```python
from build123d import *

# Parameters (mm, degrees)
BOSS_EXTRUDE1_DEPTH      = 15.875
BOSS_EXTRUDE1_DEPTH_BACK = 15.875


with BuildPart() as part:
    # Sketch2 → Boss-Extrude1 (new, two sides: drawn at the far end of the back side and taken through both)
    with BuildSketch(Plane(origin=(0, 0, 0), x_dir=(1, 0, 0), z_dir=(0, 1, 0)).offset(-BOSS_EXTRUDE1_DEPTH_BACK)):
        Polygon((-171.45, 88.9), (-171.45, -88.9), (-165.1, -88.9), (-165.1, -79.375), (-161.925, -79.375), (-161.925, 25.4), (-161.925, 34.925), (-161.925, 79.375), (-165.1, 79.375), (-165.1, 88.9), align=None)
    extrude(amount=BOSS_EXTRUDE1_DEPTH + BOSS_EXTRUDE1_DEPTH_BACK)


solid = part.part
```
Can you work these out from the model? Positions are in its coordinate system, mm. A direction names the side the tool comes from. Coordinates: 2 decimals unless noted, no trailing zeros. Loops run counter-clockwise (first coordinate to the right, second up) from the corner with the lowest first, then second, coordinate; pieces in that order, holes last.
Item 1: Please list where this line runs through material, in increasing order: L1, parallel to Z at x = -164.75, y = 4 (3 decimals).
Answers below:
L1: z = -79.375 to 79.375
Item 2: I'm going to push flat-ended pins straight in: pin 1 (1.6 mm diameter, centred on x = -163, y = 0, fed in from -Z) (3 decimals); pin 2 (1.6 mm diameter, centred on x = -164, y = -3.5, fed in from +Z) (3 decimals); pin 3 (7.5 mm diameter, centred on y = -0.5, z = -83.5, fed in from +X). Where does each tip first touch, or does it pass through?
Answers below:
pin 1: stops at z = -79.375
pin 2: stops at z = 79.375
pin 3: stops at x = -165.1
Item 3: Suppose I cut it at A-A (y = 6). Please give me the cut outline in (x, z) (3 decimals), then the cut area to 3 significant figures.
Answers below:
outline: (-171.45, -88.9) - (-165.1, -88.9) - (-165.1, -79.375) - (-161.925, -79.375) - (-161.925, 79.375) - (-165.1, 79.375) - (-165.1, 88.9) - (-171.45, 88.9) - close
area: 1,630 mm2
Item 4: Which directions (+Z, -Z, +X, -X, +Y, -Y) give clear straight access to the entire face, cutting with the end or side of a thin tool? Please do faces 1 (the face through (-168, 0, -88.9)), 2 (the face through (-164, 0, 79.375)), 3 (the face through (-165.1, 0, -84)).
Answers below:
face 1: -Z, +X, -X, +Y, -Y
face 2: +Z, +X, +Y, -Y
face 3: -Z, +X, +Y, -Y
